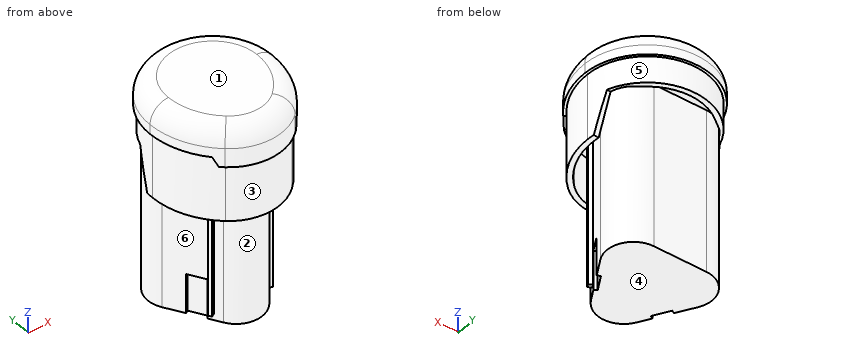
from build123d import *
from OCP.BRepFilletAPI import BRepFilletAPI_MakeChamfer

# Parameters (mm, degrees)
BOSS_EXTRU_1_DEPTH      = 80
BOSS_EXTRU_2_DEPTH      = 10.6
BOSS_EXTRU_3_DEPTH      = 10
BOSS_EXTRU_4_DEPTH      = 3.5
CHANFREIN1_SIZE         = 2
CHANFREIN1_SIZE_2       = 3.5
BOSS_EXTRU_5_DEPTH      = 14.9
CHANFREIN2_SIZE         = 5
CHANFREIN2_SIZE_2       = 14.9
ENL_V_MAT_EXTRU_1_DEPTH = 61.9
BOSS_EXTRU_8_REACH      = 92.636
BOSS_EXTRU_8_START      = -2.5
ENL_V_MAT_EXTRU_4_DEPTH = 15
CONG_1_R                = 7


with BuildPart() as part:
    # Esquisse1 → Boss.-Extru.1 (new body)
    with BuildSketch(Plane.XY):
        with BuildLine():
            Line((-9.999999999999973, 15.773502691896244), (9.999999999999973, 15.773502691896244))
            ThreePointArc((9.999999999999973, 15.773502691896244), (18.66025403784436, 10.773502691896228), (18.66025403784438, 0.7735026918962024))
            Line((18.66025403784438, 0.7735026918962024), (8.660254037844393, -16.54700538379251))
            ThreePointArc((8.660254037844393, -16.54700538379251), (-4.87e-15, -21.5470053837925), (-8.660254037844393, -16.54700538379251))
            Line((-8.660254037844393, -16.54700538379251), (-18.66025403784438, 0.7735026918962024))
            ThreePointArc((-18.66025403784438, 0.7735026918962024), (-18.66025403784441, 10.773502691896235), (-9.999999999999973, 15.773502691896244))
        make_face()
    extrude(amount=BOSS_EXTRU_1_DEPTH)

    # Esquisse2 → Boss.-Extru.2 (add)
    with BuildSketch(Plane.XY.offset(80)):
        with BuildLine():
            Line((0, 23.773502691896258), (0, -28.226497308103742))
            ThreePointArc((0, -28.226497308103742), (-7.138520611844601, -26.935621886911633), (-13.372879499304581, -23.22649730810374))
            ThreePointArc((-13.372879499304581, -23.22649730810374), (-21.14415675858487, -12.819312855059437), (-23.89999999999999, -0.12649730810374363))
            ThreePointArc((-23.89999999999999, -0.12649730810374363), (-16.89985207035848, 16.773354762254744), (0, 23.773502691896258))
        make_face()
    boss_extru_2 = extrude(amount=-BOSS_EXTRU_2_DEPTH)

    # Symétrie1: Boss.-Extru.2 across plane
    add(boss_extru_2.mirror(Plane(origin=(0, 0, 0), x_dir=(0, 0, 1), z_dir=(1, 0, 0))))

    # Esquisse4 → Boss.-Extru.3 (add)
    with BuildSketch(Plane(origin=(0, 0, 69.4), x_dir=(-1, 0, 0), z_dir=(0, 0, -1))):
        with BuildLine():
            ThreePointArc((-12.716812029717252, -22.471795065262707), (-2.04e-15, -27.226497308103735), (12.71681202971725, -22.4717950652627))
            ThreePointArc((12.71681202971725, -22.4717950652627), (20.2341931687673, -12.404624700892555), (22.899999999999995, -0.12649730810373652))
            ThreePointArc((22.899999999999995, -0.12649730810373652), (-6.91e-15, 22.773502691896258), (-22.899999999999995, -0.12649730810373735))
            ThreePointArc((-22.899999999999995, -0.12649730810373735), (-20.234193168767305, -12.404624700892553), (-12.716812029717252, -22.471795065262707))
        make_face()
    extrude(amount=BOSS_EXTRU_3_DEPTH)

    # Esquisse6 → Boss.-Extru.4 (add)
    with BuildSketch(Plane(origin=(0, 0, 69.4), x_dir=(-1, 0, 0), z_dir=(0, 0, -1))):
        with BuildLine():
            Line((14.75, -21.95321690393977), (0, -13.476497308103742))
            Line((0, -13.476497308103742), (0, -28.226497308103742))
            ThreePointArc((0, -28.226497308103742), (7.138520611844594, -26.935621886911633), (13.372879499304576, -23.226497308103735))
            ThreePointArc((13.372879499304576, -23.226497308103735), (14.071194795630928, -22.600407707254973), (14.75, -21.95321690393977))
        make_face()
    boss_extru_4 = extrude(amount=BOSS_EXTRU_4_DEPTH)

    # Symétrie2: Boss.-Extru.4 across plane
    add(boss_extru_4.mirror(Plane(origin=(0, 0, 0), x_dir=(0, 0, 1), z_dir=(1, 0, 0))))

    # Chanfrein1
    chanfrein1_edges_1 = [part.edges().sort_by_distance(p)[0] for p in [
        (-14.299309891443901, -21.69420851920438, 69.4),
    ]]
    chanfrein1_side_1 = [part.faces().sort_by_distance(p)[0] for p in [
        (-14.319240730556658, -21.659527664943543, 69.4),
    ]]
    chanfrein1_edges_2 = [part.edges().sort_by_distance(p)[0] for p in [
        (14.299309891443906, -21.694208519204384, 69.4),
    ]]
    chanfrein1_side_2 = [part.faces().sort_by_distance(p)[0] for p in [
        (14.319240730556663, -21.659527664943546, 69.4),
    ]]
    chanfrein1 = BRepFilletAPI_MakeChamfer(part.part.solid().wrapped)
    for e in chanfrein1_edges_1:
        chanfrein1.Add(CHANFREIN1_SIZE - 0.0001, CHANFREIN1_SIZE_2 - 0.0001, e.wrapped, chanfrein1_side_1[0].wrapped)
    for e in chanfrein1_edges_2:
        chanfrein1.Add(CHANFREIN1_SIZE - 0.0001, CHANFREIN1_SIZE_2 - 0.0001, e.wrapped, chanfrein1_side_2[0].wrapped)
    add(Compound.cast(chanfrein1.Shape()), mode=Mode.REPLACE)  # a hair under: the kernel refuses the full size

    # Esquisse7 → Boss.-Extru.5 (add)
    with BuildSketch(Plane(origin=(0, 0, 59.4), x_dir=(-1, 0, 0), z_dir=(0, 0, -1))):
        with BuildLine():
            Line((-6.79e-15, -27.22649730810374), (0, 0))
            Line((0, 0), (22.71563338320109, 2.7735026918962267))
            ThreePointArc((22.71563338320109, 2.7735026918962267), (22.853861867037974, 1.3264299999015228), (22.899999999999995, -0.12649730810374016))
            ThreePointArc((22.899999999999995, -0.12649730810374016), (20.2341931687673, -12.404624700892562), (12.716812029717245, -22.471795065262707))
            ThreePointArc((12.716812029717245, -22.471795065262707), (6.788307992740876, -25.998951656029643), (-6.79e-15, -27.22649730810374))
        make_face()
    boss_extru_5 = extrude(amount=BOSS_EXTRU_5_DEPTH)

    # Symétrie4: Boss.-Extru.5 across plane
    add(boss_extru_5.mirror(Plane(origin=(0, 0, 0), x_dir=(0, 0, 1), z_dir=(1, 0, 0))))

    # Chanfrein2
    chanfrein2_edges_1 = [part.edges().sort_by_distance(p)[0] for p in [
        (21.059128460282075, 2.5712489935136453, 59.4),
    ]]
    chanfrein2_side_1 = [part.faces().sort_by_distance(p)[0] for p in [
        (21.04700879877706, 2.6705118456034573, 59.4),
    ]]
    chanfrein2_edges_2 = [part.edges().sort_by_distance(p)[0] for p in [
        (-21.059128460282082, 2.571248993513646, 59.4),
    ]]
    chanfrein2_side_2 = [part.faces().sort_by_distance(p)[0] for p in [
        (-21.059128460282082, 2.571248993513646, 59.3),
    ]]
    chanfrein2 = BRepFilletAPI_MakeChamfer(part.part.solid().wrapped)
    for e in chanfrein2_edges_1:
        chanfrein2.Add(CHANFREIN2_SIZE - 0.0001, CHANFREIN2_SIZE_2 - 0.0001, e.wrapped, chanfrein2_side_1[0].wrapped)
    for e in chanfrein2_edges_2:
        chanfrein2.Add(CHANFREIN2_SIZE_2 - 0.0001, CHANFREIN2_SIZE - 0.0001, e.wrapped, chanfrein2_side_2[0].wrapped)
    add(Compound.cast(chanfrein2.Shape()), mode=Mode.REPLACE)  # a hair under: the kernel refuses the full size

    # Esquisse8 → Enlèv. mat.-Extru.1 (cut)
    with BuildSketch(Plane(origin=(0, 0, 0), x_dir=(-1, 0, 0), z_dir=(0, 0, -1))):
        with BuildLine():
            Line((-20.73173527113113, 2.5202275827259273), (-20.108299540895768, 7.138156637600371))
            ThreePointArc((-20.108299540895768, 7.138156637600371), (-18.785258977060302, 10.95609130242486), (-16.08354229758742, 13.96071913666333))
            Line((-16.08354229758742, 13.96071913666333), (-12.465297452899778, 16.64926972087978))
            ThreePointArc((-12.465297452899778, 16.64926972087978), (8.34e-15, 20.773502691896244), (12.465297452899788, 16.649269720879765))
            Line((12.465297452899788, 16.649269720879765), (16.083542297587456, 13.96071913666329))
            ThreePointArc((16.083542297587456, 13.96071913666329), (18.78525897706036, 10.956091302424788), (20.108299540895814, 7.13815663760026))
            Line((20.108299540895814, 7.13815663760026), (20.73173527113112, 2.5202275827259264))
            ThreePointArc((20.73173527113112, 2.5202275827259264), (20.857891398301028, 1.1995367852285772), (20.89999999999999, -0.12649730810373677))
            ThreePointArc((20.89999999999999, -0.12649730810373677), (18.414265989132176, -11.5752483925588), (11.404677090542576, -20.962390579580656))
            ThreePointArc((11.404677090542576, -20.962390579580656), (1.69e-15, -25.226497308103735), (-11.40467709054258, -20.962390579580664))
            ThreePointArc((-11.40467709054258, -20.962390579580664), (-18.414265989132176, -11.575248392558798), (-20.89999999999999, -0.1264973081037376))
            ThreePointArc((-20.89999999999999, -0.1264973081037376), (-20.85789139830103, 1.1995367852285768), (-20.73173527113113, 2.5202275827259273))
        make_face()
        with BuildLine():
            Line((-18.66025403784436, 0.773502691896218), (-8.660254037844393, -16.54700538379251))
            ThreePointArc((-8.660254037844393, -16.54700538379251), (6.09e-15, -21.547005383792524), (8.660254037844393, -16.54700538379251))
            Line((8.660254037844393, -16.54700538379251), (18.66025403784438, 0.7735026918962024))
            ThreePointArc((18.66025403784438, 0.7735026918962024), (18.66025403784438, 10.773502691896217), (9.999999999999973, 15.773502691896226))
            Line((9.999999999999973, 15.773502691896226), (-9.999999999999973, 15.773502691896244))
            ThreePointArc((-9.999999999999973, 15.773502691896244), (-18.660254037844357, 10.77350269189623), (-18.66025403784436, 0.773502691896218))
        make_face(mode=Mode.SUBTRACT)
    extrude(amount=-ENL_V_MAT_EXTRU_1_DEPTH, mode=Mode.SUBTRACT)

    # Esquisse9 → Boss.-Extru.8 (add, up to next)
    with BuildSketch(Plane(origin=(0, 0, 0), x_dir=(-1, 0, 0), z_dir=(0, 0, -1)).offset(BOSS_EXTRU_8_START), mode=Mode.PRIVATE) as boss_extru_8_sk1:
        Polygon((-10.214359353944898, -13.855216015993522), (-11.599999999999998, -14.655216015993522), (-12.3, -13.442780450695311), (-10.914359353944906, -12.642780450695314), align=None)
    boss_extru_8_tool1 = extrude(boss_extru_8_sk1.sketch, amount=-BOSS_EXTRU_8_REACH, mode=Mode.PRIVATE) - part.part
    # Esquisse9 → Boss.-Extru.8 (add, up to next)
    with BuildSketch(Plane(origin=(0, 0, 0), x_dir=(-1, 0, 0), z_dir=(0, 0, -1)).offset(BOSS_EXTRU_8_START), mode=Mode.PRIVATE) as boss_extru_8_sk2:
        Polygon((10.914359353944906, -12.642780450695314), (10.214359353944898, -13.855216015993522), (11.599999999999998, -14.655216015993522), (12.3, -13.442780450695311), align=None)
    boss_extru_8_tool2 = extrude(boss_extru_8_sk2.sketch, amount=-BOSS_EXTRU_8_REACH, mode=Mode.PRIVATE) - part.part
    add(boss_extru_8_tool1.solids().sort_by_distance((11.25718, -13.648998, 2.5))[0])
    add(boss_extru_8_tool2.solids().sort_by_distance((-11.25718, -13.648998, 2.5))[0])

    # Esquisse10 → Enlèv. mat.-Extru.4 (cut)
    with BuildSketch(Plane(origin=(0, 0, 0), x_dir=(-1, 0, 0), z_dir=(0, 0, -1))):
        Polygon((-11.249999999999988, -12.061433798642668), (-10.124166975080218, -11.411433798642664), (-13.624166975080218, -5.349255972151593), (-14.74999999999999, -5.999255972151601), align=None)
        Polygon((11.250000000000012, -12.061433798642668), (14.750000000000009, -5.9992559721515955), (13.624166975080241, -5.349255972151597), (10.124166975080241, -11.411433798642667), align=None)
    extrude(amount=-ENL_V_MAT_EXTRU_4_DEPTH, mode=Mode.SUBTRACT)

    # Congé1
    cong_1_edges = [part.edges().sort_by_distance(p)[0] for p in [
        (-1.79e-15, 23.773502691896258, 80),
        (-21.144156758584863, -12.819312855059447, 80),
        (6.22e-15, -28.226497308103745, 80),
        (21.144156758584863, -12.819312855059447, 80),
    ]]
    fillet(cong_1_edges, radius=CONG_1_R)


solid = part.part
Build history of the part. All positions in model axes, mm. Face numbers are marked on the shaded views. A direction names the side the tool comes from. Round coordinates to 2 decimals unless told otherwise and drop trailing zeros. Write each loop counter-clockwise with the first axis right and the second up, starting at its lowest first coordinate (ties: lowest second). Pieces come first, ordered by that corner, then holes. Notation, with made-up numbers: M -20,-28 L 14,-28 A27 ccw 14,1 Z; hole C 22.5,-22 d6. An arc over 180 degrees is marked long. Answer as a JSON object with one key per item and string values. Group by question number.
(1) Cut at A-A (x = 0). Give the cut face in (y, z), and give its area (3 significant figures).
(2) Drill centre lines: L1, parallel to Y at x = -11, z = 50; L2, parallel to X at y = 6, z = 18; L3, parallel to X at y = 2, z = 54.5. Where is each one in solid material? Low to high.
(3) Flat gauge pins, fed straight in: pin 1 (12 mm diameter, centred on x = -5, z = 35, fed in from -Y); pin 2 (12 mm diameter, centred on x = -8.5, z = 8.5, fed in from +Y); pin 3 (5 mm diameter, centred on x = -15, z = 26.5, fed in from -Y). Where does each tip first touch, or does it go through?
(4) Which spindle directions (+Z, -Z, +X, -X, +Y, -Y) get a long thin tool onto all of the face, cutting with end or side? Do the marked faces 1, 2 and 3. Say none if no direction does.
(5) Mould opens along X. For the marked faces 4, 5 and 6 say: pulls with the +X half, pulls with the -X half, needs draft (parallel to the pull), parting line crosses it, or undercut.
(6) Cut at C-C (z = 46.5). Give the cut face in (x, y), and give its area (3 significant figures).
(7) Cut at B-B (z = 31). Give the cut face in (x, y).
Responses:
{
 "1": {"outline": "M -28.23,65.9 L -27.23,65.9 L -27.23,44.5 L -25.23,44.5 L -25.23,61.9 L -21.55,61.9 L -21.55,0 L 15.77,0 L 15.77,61.9 L 20.77,61.9 L 20.77,59.4 L 22.77,59.4 L 22.77,69.4 L 23.77,69.4 L 23.77,73 A7 ccw 16.77,80 L -21.23,80 A7 ccw -28.23,73 Z", "area": "3,260 mm2"},
 "2": {"L1": "y = -23.8 to -21.3, -14.31 to -12.69, -12.49 to 15.72", "L2": "x = -20 to 20", "L3": "x = -22.8 to -20.79, -19.26 to 19.26, 20.79 to 22.8"},
 "3": {"pin 1": "stops at y = -21.55", "pin 2": "stops at y = 15.77", "pin 3": "stops at y = -9.9"},
 "4": {"face 1": "+Z, +X, -X, +Y, -Y", "face 2": "-Z", "face 3": "-Z, -Y"},
 "5": {"face 4": "needs draft", "face 5": "parting line crosses it", "face 6": "undercut"},
 "6": {"outline": "M -22.9,-0.13 A29.61 ccw -12.72,-22.47 A19.38 ccw 12.72,-22.47 A29.61 ccw 22.9,-0.13 A22.9 ccw 22.62,3.44 L 20.64,3.2 L 20.73,2.52 A20.9 cw 20.9,-0.13 A27.61 cw 11.4,-20.96 A17.38 cw -11.4,-20.96 A27.61 cw -20.9,-0.13 A20.9 cw -20.73,2.52 L -20.64,3.2 L -22.62,3.44 A22.9 ccw Z; M -18.66,0.77 L -10.91,-12.64 L -12.3,-13.44 L -11.6,-14.66 L -10.21,-13.86 L -8.66,-16.55 A10 ccw 8.66,-16.55 L 10.21,-13.86 L 11.6,-14.66 L 12.3,-13.44 L 10.91,-12.64 L 18.66,0.77 A10 ccw 10,15.77 L -10,15.77 A10 ccw Z", "area": "1,260 mm2"},
 "7": {"outline": "M -18.66,0.77 L -10.91,-12.64 L -12.3,-13.44 L -11.6,-14.66 L -10.21,-13.86 L -8.66,-16.55 A10 ccw 8.66,-16.55 L 10.21,-13.86 L 11.6,-14.66 L 12.3,-13.44 L 10.91,-12.64 L 18.66,0.77 A10 ccw 10,15.77 L -10,15.77 A10 ccw Z"}
}
